from build123d import *

# Parameters (mm, degrees)
SKETCH005_R             = 15.9
PAD003_DEPTH            = 4.8
SKETCH004_R             = 12.5
PAD002_DEPTH            = 9
CHAMFER002_SIZE         = 0.7
BODY001_PLACEMENT_ANGLE = 90


with BuildPart() as part:
    # Sketch005 → Pad003 (new body)
    with BuildSketch(Plane.XY):
        Circle(SKETCH005_R)
    extrude(amount=PAD003_DEPTH)

    # Sketch004 (on Face3 of Pad003) → Pad002 (join)
    with BuildSketch(Plane.XY.offset(4.8)):
        Circle(SKETCH004_R)
    extrude(amount=PAD002_DEPTH)

    # Chamfer002
    chamfer002_edges = [part.edges().sort_by_distance(p)[0] for p in [
        (-12.5, 0, 13.8),
    ]]
    chamfer(chamfer002_edges, length=CHAMFER002_SIZE)


with BuildPart() as part_1:
    # Body001 placement: moved
    add(part.part.moved(Location((0, -60, -4.5))).rotate(Axis((0, -60, -4.5), (-1, 0, 0)), BODY001_PLACEMENT_ANGLE))


solid = part_1.part
Read the model definition and answer for the solid it produces. Units are mm, in the model's axes. A direction names the side the tool comes from. Coordinates: 2 decimals unless noted, no trailing zeros. Order: outer loops, then holes, each group sorted by start corner. A loop starts at its lowest first (then second) coordinate and runs counter-clockwise, first axis right, second up. Notation, with made-up numbers: M 76.5,70.25 L 103.5,70.25 A8 ccw 103.5,81.25 Z; hole C -38,80.5 d5. An arc over 180 degrees is marked long. Put each result on its own line as item: value. Start each with the question number.
Item 1: Section B-B, the plane x = 0 is taken. Determine the outline of the cut face in (y, z).
Item 2: For faces 1 (the face through (-11, -55.2, 2)), 2 (the face through (0, -46.2, -5)), determine the directions among +Z, -Z, +X, -X, +Y, -Y from which every point of the face is accessible in a straight line to the end or side of a thin tool.
Item 3: Given pin 1 Ø5 at (y, z) = (-51, 7) entering from +X; pin 2 Ø3 at (x, y) = (3, -50) entering from -Z; pin 3 Ø6 at (x, z) = (-11.5, 6.5) entering from +Y, each flat-ended and moving along its own axis, determine where each tip first touches the part or whether it passes through.
Item 4: Consider probe 1 along Y at (x, z) = (10, 7.5); probe 2 along X at (y, z) = (-52.5, -4); probe 3 along X at (y, z) = (-48.5, 2). Determine where each line is inside the solid, lowest interval first. Write a range as [from, to].
Item 5: Section D-D, the plane y = -58.5 is taken. Determine the outline of the cut face in (x, z).
Item 6: Section A-A, the plane z = -4.5 is taken. Determine the outline of the cut face in (x, y), plus the area to 3 significant figures.
Item 7: Section C-C, the plane y = -48.25 is taken. Determine the outline of the cut face in (x, z).
Computed:
1. outline: M -60,-20.4 L -55.2,-20.4 L -55.2,-17 L -46.9,-17 L -46.2,-16.3 L -46.2,7.3 L -46.9,8 L -55.2,8 L -55.2,11.4 L -60,11.4 Z
2. face 1: +Y
2. face 2: +Z, -Z, +X, -X, +Y
3. pin 1: stops at x = 8.67
3. pin 2: stops at z = -16.91
3. pin 3: stops at y = -55.2
4. probe 1: y = [-60, -55.2]
4. probe 2: x = [-12.49, 12.49]
4. probe 3: x = [-10.68, 10.68]
5. outline: C 0,-4.5 d31.8
6. outline: M -15.9,-60 L 15.9,-60 L 15.9,-55.2 L 12.5,-55.2 L 12.5,-46.9 L 11.8,-46.2 L -11.8,-46.2 L -12.5,-46.9 L -12.5,-55.2 L -15.9,-55.2 Z
6. area: 377 mm2
7. outline: C 0,-4.5 d25
